Verification items for the finished model (mm, model axes). A direction names the side the tool comes from. Round coordinates to 2 decimals unless told otherwise and drop trailing zeros. Write each loop counter-clockwise with the first axis right and the second up, starting at its lowest first coordinate (ties: lowest second). Pieces come first, ordered by that corner, then holes. Notation, with made-up numbers: (36, -11) -> (89, -11) arc R20 cw to (89, 14) -> close; hole circle Ø1 at (13.5, -17). An arc over 180 degrees is marked (long way). Answer as a JSON object with one key per item and string values. Group by question number.
(1) Gauge pin test, flat ends, axial feed: pin 1 Ø4 at (x, z) = (3.5, -1.5) entering from +Y; pin 2 Ø1.5 at (x, z) = (-6, -4.5) entering from -Y; pin 3 Ø4 at (x, y) = (-3.1, 5.37) entering from -Z; pin 4 Ø3 at (y, z) = (-4.5, 1) entering from -X. Record the tip position at first contact, or that the pin passes through.
(2) Sectioned sample at A-A on y = 0. Record the cut outline in (x, z), and give its area (3 significant figures).
(3) Sectioned sample at D-D on x = -3.1. Count the separate pieces of the cut face and the enclosed holes in it, and give its area (3 significant figures).
(4) Sectioned sample at C-C on z = -5.25. Record the cut outline in (x, y).
(5) Draft check along X on faces 3 (the face through (0, 3, -6.4)), 4 (the face through (7.63, 0.45, 1.48)), 5 (the face through (0.867, -3.905, -3.159)). Enter one of: released by +X, released by -X, zero draft, split by the parting line, or undercut.
(6) Scan lines: L1, parallel to Y at x = -3.1, z = 2.1; L2, parallel to Z at x = 5.25, y = 6.75; L3, parallel to Y at x = 6.2, z = 0.7. Record each from-to range of solid material in increasing order. Write a range as from..to.
(7) Set-up check for faces 1 (the face through (4, -2, 0)), 2 (the face through (2, -2, 3)): record each of +Z, -Z, +X, -X, +Y, -Y from which the full face is reachable in a straight line by a thin tool's end or side.
(8) Sectioned sample at B-B on x = 0. Record the cut outline in (y, z), and give its area (3 significant figures).
```python
from build123d import *

# Parameters (mm, degrees)
SKETCH1_R           = 10
SKETCH1_R_2         = 2.5
SKETCH1_R_3         = 1.5
BOSS_EXTRUDE1_DEPTH = 3
SKETCH2_R           = 4
SKETCH2_R_2         = 2.5
BOSS_EXTRUDE2_DEPTH = 6.4
FILLET1_R           = 0.25
FILLET2_R           = 0.25
FILLET3_R           = 0.25


with BuildPart() as part:
    # Sketch1 → Boss-Extrude1 (new body)
    with BuildSketch(Plane.XY):
        Circle(SKETCH1_R)
        Circle(SKETCH1_R_2, mode=Mode.SUBTRACT)
        with Locations((6.2, 0)):
            Circle(SKETCH1_R_3, mode=Mode.SUBTRACT)
        with Locations((-3.1, -5.369357503)):
            Circle(SKETCH1_R_3, mode=Mode.SUBTRACT)
        with Locations((-3.1, 5.369357503)):
            Circle(SKETCH1_R_3, mode=Mode.SUBTRACT)
    extrude(amount=BOSS_EXTRUDE1_DEPTH)

    # Sketch2 → Boss-Extrude2 (add)
    with BuildSketch(Plane(origin=(0, 0, 0), x_dir=(-1, 0, 0), z_dir=(0, 0, -1))):
        Circle(SKETCH2_R)
        Circle(SKETCH2_R_2, mode=Mode.SUBTRACT)
    extrude(amount=BOSS_EXTRUDE2_DEPTH)

    # Fillet1
    fillet1_edges = [part.edges().sort_by_distance(p)[0] for p in [
        (4, 0, 0),
    ]]
    fillet(fillet1_edges, radius=FILLET1_R)

    # Fillet2
    fillet2_edges = [part.edges().sort_by_distance(p)[0] for p in [
        (4, 0, -6.4),
    ]]
    fillet(fillet2_edges, radius=FILLET2_R)

    # Fillet3
    fillet3_edges = [part.edges().sort_by_distance(p)[0] for p in [
        (-10, 0, 0),
        (-10, 0, 3),
    ]]
    fillet(fillet3_edges, radius=FILLET3_R)


solid = part.part
```
Computed values:
{
 "1": {"pin 1": "y = 9.69", "pin 2": "through", "pin 3": "z = 0", "pin 4": "x = -9.54"},
 "2": {"outline": "(-10, 0.25) arc R0.25 ccw to (-9.75, 0) -> (-4.25, 0) arc R0.25 cw to (-4, -0.25) -> (-4, -6.15) arc R0.25 ccw to (-3.75, -6.4) -> (-2.5, -6.4) -> (-2.5, 3) -> (-9.75, 3) arc R0.25 ccw to (-10, 2.75) -> close; (2.5, -6.4) -> (3.75, -6.4) arc R0.25 ccw to (4, -6.15) -> (4, -0.25) arc R0.25 cw to (4.25, 0) -> (4.7, 0) -> (4.7, 3) -> (2.5, 3) -> close; (7.7, 0) -> (9.75, 0) arc R0.25 ccw to (10, 0.25) -> (10, 2.75) arc R0.25 ccw to (9.75, 3) -> (7.7, 3) -> close", "area": "55.1 mm2"},
 "3": {"separate pieces": "3", "enclosed holes": "0", "area": "71.3 mm2"},
 "4": {"outline": "circle Ø8 at (0, 0); hole circle Ø5 at (0, 0)"},
 "5": {"face 3": "zero draft", "face 4": "undercut", "face 5": "split by the parting line"},
 "6": {"L1": "-9.51..-6.87, -3.87..3.87, 6.87..9.51", "L2": "0..3", "L3": "-7.85..-1.5, 1.5..7.85"},
 "7": {"face 1": "-Z", "face 2": "+Z, +X, -X, +Y, -Y"},
 "8": {"outline": "(-10, 0.25) arc R0.25 ccw to (-9.75, 0) -> (-4.25, 0) arc R0.25 cw to (-4, -0.25) -> (-4, -6.15) arc R0.25 ccw to (-3.75, -6.4) -> (-2.5, -6.4) -> (-2.5, 3) -> (-9.75, 3) arc R0.25 ccw to (-10, 2.75) -> close; (2.5, -6.4) -> (3.75, -6.4) arc R0.25 ccw to (4, -6.15) -> (4, -0.25) arc R0.25 cw to (4.25, 0) -> (9.75, 0) arc R0.25 ccw to (10, 0.25) -> (10, 2.75) arc R0.25 ccw to (9.75, 3) -> (2.5, 3) -> close", "area": "64.1 mm2"}
}
